Study the drawing (mm; zero at the part's minimum x, y, z) and answer. A direction names the side the tool comes from. Give positions to 0.01 mm unless a question says otherwise; leave off trailing zeros. Order: outer loops, then holes, each group sorted by start corner. A loop starts at its lowest first (then second) coordinate and runs counter-clockwise, first axis right, second up.
Item 1: Given pin 1 Ø1.5 at (x, y) = (24, 4) entering from -Z, flat-ended and moving along its own axis, determine where the tip first touches the part or whether it passes through.
Item 2: Find the intervals of material crossed by line 1 along X through (y, z) = (5.5, 4); line 2 along Y through (x, z) = (11, 1.45); line 3 along Z through (x, y) = (18, 8), in increasing order.
Item 3: A cutting plane is placed at B-B (y = 6). Write down the section's boundary in (x, z), plus the area to 3 significant figures.
Item 4: A cutting plane is placed at D-D (z = 8). Write down the section's boundary in (x, y), plus the area to 3 significant figures.
Item 5: A cutting plane is placed at A-A (z = 4.25). Write down the section's boundary in (x, y).
Item 6: Which of the six approach directions +Z, -Z, +X, -X, +Y, -Y give full straight-line access (tool end or side, diameter ignored) to the marked faces 4, 5 and 6?
Item 7: The mould has two halves that part along X. Classify the marked faces 1, 2 and 3: +X half, -X half, draft (parallel to the pull), parting line (faces both ways), or undercut.
Item 8: A cutting plane is placed at C-C (x = 27). Write down the section's boundary in (y, z), plus the area to 3 significant figures.
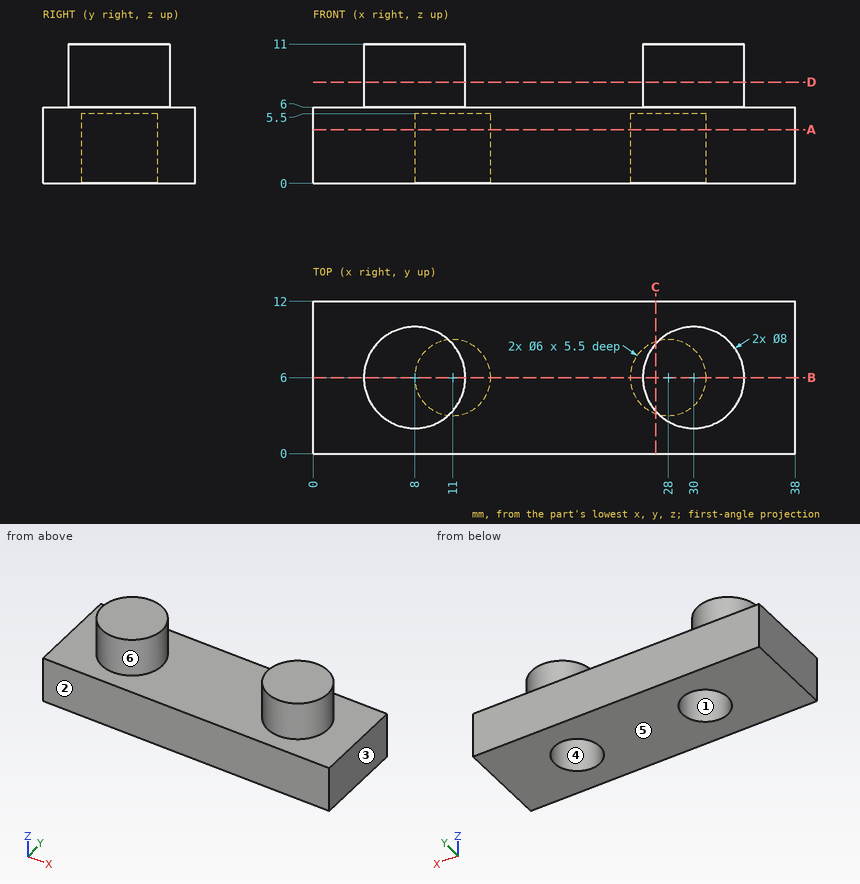
Response values:
1. pin 1: stops at z = 0
2. line 1: x = 0 to 8.04, 13.96 to 25.04, 30.96 to 38
2. line 2: y = 0 to 3, 9 to 12
2. line 3: z = 0 to 6
3. outline: (0, 0) - (8, 0) - (8, 5.5) - (14, 5.5) - (14, 0) - (25, 0) - (25, 5.5) - (31, 5.5) - (31, 0) - (38, 0) - (38, 6) - (34, 6) - (34, 11) - (26, 11) - (26, 6) - (12, 6) - (12, 11) - (4, 11) - (4, 6) - (0, 6) - close
3. area: 242 mm2
4. outline: circle Ø8 at (8, 6); circle Ø8 at (30, 6)
4. area: 101 mm2
5. outline: (0, 0) - (38, 0) - (38, 12) - (0, 12) - close; hole circle Ø6 at (11, 6); hole circle Ø6 at (28, 6)
6. face 4: -Z
6. face 5: -Z, +X, -X, +Y, -Y
6. face 6: +Z
7. face 1: undercut
7. face 2: draft
7. face 3: +X half
8. outline: (0, 0) - (3.17, 0) - (3.17, 5.5) - (8.83, 5.5) - (8.83, 0) - (12, 0) - (12, 6) - (8.65, 6) - (8.65, 11) - (3.35, 11) - (3.35, 6) - (0, 6) - close
8. area: 67.3 mm2
